```python
from build123d import *

# Parameters (mm, degrees)
BOSS_EXTRUDE1_DEPTH = 2.7
BOSS_EXTRUDE2_DEPTH = 2
BOSS_EXTRUDE3_DEPTH = 2.5
SKETCH9_W           = 60
SKETCH9_H           = 5
CUT_EXTRUDE6_DEPTH  = 10
SKETCH11_W          = 25.492902138
SKETCH11_H          = 3.302010066
SKETCH11_W_2        = 3.620048782
SKETCH11_H_2        = 15.848017525
SKETCH11_W_3        = 3.810768748
SKETCH11_H_3        = 15.769779212
CUT_EXTRUDE7_DEPTH  = 4.5


with BuildPart() as part:
    # Sketch1 → Boss-Extrude1 (new body)
    with BuildSketch(Plane.XY):
        Polygon((-54.373493976, 36.84753086), (-63.373493976, 36.84753086), (-63.373493976, -23.15246914), (-3.373493976, -23.15246914), (-3.373493976, 36.84753086), (-12.373493976, 36.84753086), (-12.373493976, -13.15246914), (-54.373493976, -13.15246914), align=None)
    extrude(amount=BOSS_EXTRUDE1_DEPTH)

    # Sketch3 → Boss-Extrude2 (add)
    with BuildSketch(Plane(origin=(0, 0, 0), x_dir=(-1, 0, 0), z_dir=(0, 0, -1))):
        Polygon((9.373493976, -16.15246914), (9.373493976, 36.84753086), (5.373493976, 36.84753086), (5.373493976, -20.15246914), (61.373493976, -20.15246914), (61.373493976, 36.84753086), (57.373493976, 36.84753086), (57.373493976, -16.15246914), align=None)
    extrude(amount=BOSS_EXTRUDE2_DEPTH)

    # Sketch4 → Boss-Extrude3 (add)
    with BuildSketch(Plane(origin=(0, 0, -2), x_dir=(-1, 0, 0), z_dir=(0, 0, -1))):
        Polygon((55.373493976, 36.84753086), (55.373493976, -14.15246914), (11.373493976, -14.15246914), (11.373493976, 36.84753086), (5.373493976, 36.84753086), (5.373493976, -20.15246914), (61.373493976, -20.15246914), (61.373493976, 36.84753086), align=None)
    extrude(amount=BOSS_EXTRUDE3_DEPTH)

    # Sweep1: sweep along a curve in space
    with BuildLine() as sweep1_path:
        Line((-33.373493976, -20.65246914, 0), (-33.373493976, -19.954479206, -19.98781654))
    # Sketch9 → Sweep1 (sweep)
    with BuildSketch(Plane(origin=(0, 0, 0), x_dir=(-1, 0, 0), z_dir=(0, 0, -1))):
        with Locations((33.373493976, -20.65246914)):
            Rectangle(SKETCH9_W, SKETCH9_H)
    sweep(path=sweep1_path.line)

    # Sketch10 → Cut-Extrude6 (cut)
    with BuildSketch(Plane(origin=(0, 0, -4.5), x_dir=(-1, 0, 0), z_dir=(0, 0, -1))):
        Polygon((3.373493976, 7.545520794), (63.373493976, 7.545520794), (73.535080065, 7.545520794), (73.535080065, 46.239057039), (-7.104014128, 46.239057039), (-7.104014128, 7.545520794), align=None)
    extrude(amount=-CUT_EXTRUDE6_DEPTH, mode=Mode.SUBTRACT)

    # Sketch11 → Cut-Extrude7 (cut)
    with BuildSketch(Plane(origin=(0, 0, -4.5), x_dir=(-1, 0, 0), z_dir=(0, 0, -1))):
        with Locations((33.405280637, -15.803474173)):
            Rectangle(SKETCH11_W, SKETCH11_H)
        with Locations((9.563469585, -3.743911731)):
            Rectangle(SKETCH11_W_2, SKETCH11_H_2)
        with Locations((57.27887835, -3.704792574)):
            Rectangle(SKETCH11_W_3, SKETCH11_H_3)
    extrude(amount=-CUT_EXTRUDE7_DEPTH, mode=Mode.SUBTRACT)


solid = part.part
```
Design review of the part built by this model. Coordinates are the model's own, in mm. A direction names the side the tool comes from. Coordinates: 2 decimals unless noted, no trailing zeros. Order: outer loops, then holes, each group sorted by start corner. A loop starts at its lowest first (then second) coordinate and runs counter-clockwise, first axis right, second up.
1) Take a section at A-A, the plane y = -10.5. Give the boundary of the cut face in (x, z), and give its area (3 significant figures).
2) Mouldability with a two-part tool opening along Z and no side actions: class faces 4 (the flat face through (-34, -14, 2.7)), 5 (the flat face through (-52, -16.152, -1)), 6 (the flat face through (-33, -17.454, -2)) as +Z half, -Z half, draft (parallel to the pull), parting line (faces both ways), or undercut.
3) Take a section at D-D, the plane x = -41. Give the boundary of the cut face in (y, z), and give its area (3 significant figures).
4) For faces 1 (the flat face through (-11.373, 6, -3)), 2 (the flat face through (-58, -11.59, -3)), 3 (the flat face through (-57.373, -14, -1)), list the 3-axis set-ups (+Z, -Z, +X, -X, +Y, -Y) from which the entire face can be reached by the end or side of a thin tool; tool diameter is ignored.
5) Take a section at B-B, the plane x = -52.5. Give the boundary of the cut face in (y, z).
6) Wall thickness on line 1 along Z through (x, y) = (-51.5, -16); line 2 along X through (y, z) = (-0.5, 1); line 3 along Z through (x, y) = (-8.5, 5): over which ranges is each line inside the solid? List them lowest first.
7) Take a section at C-C, the plane z = 1. Give the boundary of the cut face in (x, y), and give its area (3 significant figures).
8) Clearance check with flat-ended pins moving along their axes: pin 1 (0.6 mm diameter, centred on x = -54, z = -1, fed in from +Y); pin 2 (3.5 mm diameter, centred on y = -1, z = -3, fed in from -X); pin 3 (0.6 mm diameter, centred on x = -62.5, y = -3, fed in from -Z). State where each tip first meets the part, or that it passes through.
Returned:
1. outline: (-63.37, 0) - (-61.37, 0) - (-61.37, -4.5) - (-59.18, -4.5) - (-59.18, 0) - (-54.37, 0) - (-54.37, 2.7) - (-63.37, 2.7) - close; (-12.37, 0) - (-7.75, 0) - (-7.75, -4.5) - (-5.37, -4.5) - (-5.37, 0) - (-3.37, 0) - (-3.37, 2.7) - (-12.37, 2.7) - close
1. area: 69.2 mm2
2. face 4: +Z half
2. face 5: undercut
2. face 6: draft
3. outline: (-23.15, 0) - (-22.45, -19.99) - (-17.45, -19.99) - (-18, -4.5) - (-17.45, -4.5) - (-17.45, 0) - (-13.15, 0) - (-13.15, 2.7) - (-23.15, 2.7) - close
3. area: 130 mm2
4. face 1: -Z, +Y
4. face 2: -Z
4. face 3: +Y
5. outline: (-23.15, 0) - (-22.45, -19.99) - (-17.45, -19.99) - (-18, -4.5) - (-14.15, -4.5) - (-14.15, -2) - (-16.15, -2) - (-16.15, 0) - (-13.15, 0) - (-13.15, 2.7) - (-23.15, 2.7) - close
6. line 1: z = -4.5 to -2, 0 to 2.7
6. line 2: x = -63.37 to -54.37, -12.37 to -3.37
6. line 3: z = -4.5 to 2.7
7. outline: (-63.37, -23.15) - (-3.37, -23.15) - (-3.37, 7.55) - (-12.37, 7.55) - (-12.37, -13.15) - (-54.37, -13.15) - (-54.37, 7.55) - (-63.37, 7.55) - close
7. area: 973 mm2
8. pin 1: stops at y = -16.15
8. pin 2: stops at x = -61.37
8. pin 3: stops at z = 0
